from build123d import *

# Parameters (mm, degrees)
SKETCH010_W      = 209.545
SKETCH010_H      = 125
SKETCH010_R      = 1.6
EXTRUDE010_DEPTH = 1.6
SKETCH015_W      = 28
SKETCH015_H      = 8.6
EXTRUDE014_DEPTH = 10


with BuildPart() as extrude010:
    # Sketch010 → Extrude010 (new body)
    with BuildSketch(Plane.XY.offset(38)):
        with Locations((192.2275, 147.5)):
            Rectangle(SKETCH010_W, SKETCH010_H)
        with Locations((93.455, 204)):
            Circle(SKETCH010_R, mode=Mode.SUBTRACT)
        with Locations((291, 204)):
            Circle(SKETCH010_R, mode=Mode.SUBTRACT)
        with Locations((291, 91)):
            Circle(SKETCH010_R, mode=Mode.SUBTRACT)
        with Locations((93.455, 91)):
            Circle(SKETCH010_R, mode=Mode.SUBTRACT)
    extrude(amount=EXTRUDE010_DEPTH)


with BuildPart() as rf16:
    # Sketch015 (on Face10 of Extrude010) → Extrude014 (new body)
    with BuildSketch(Plane.XY.offset(39.6)):
        with Locations((272.87, 107.23)):
            Rectangle(SKETCH015_W, SKETCH015_H)
        with Locations((272.87, 117.39)):
            Rectangle(SKETCH015_W, SKETCH015_H)
        with Locations((208.11, 198.57)):
            Rectangle(SKETCH015_W, SKETCH015_H)
        with Locations((178.9, 198.57)):
            Rectangle(SKETCH015_W, SKETCH015_H)
        with Locations((149.69, 198.57)):
            Rectangle(SKETCH015_W, SKETCH015_H)
        with Locations((120.48, 198.57)):
            Rectangle(SKETCH015_W, SKETCH015_H)
    extrude(amount=EXTRUDE014_DEPTH)

    # Fusion005: union Extrude010
    add(extrude010.part)


solid = rf16.part
Source: CAD feature listing. Evaluate the final solid. Frame: model axes, mm. A direction names the side the tool comes from. Give positions to 0.01 mm unless a question says otherwise; leave off trailing zeros. Order: outer loops, then holes, each group sorted by start corner. A loop starts at its lowest first (then second) coordinate and runs counter-clockwise, first axis right, second up. Notation, with made-up numbers: (37.25, -20.5) -> (51.25, -20.5) arc R23 ccw to (51.25, 8.5) -> close; hole circle Ø3 at (88.25, -18.75). An arc over 180 degrees is marked (long way). Use a Markdown table: item, result.
1) Ray query, line 1 along X through (y, z) = (204, 38.4) (3 decimals); line 2 along X through (y, z) = (197.5, 43); line 3 along Y through (x, z) = (291, 38.75). Return the intervals inside material, ascending. Write a range as [from, to].
Answer list:
| item | result |
|---|---|
| line 1 | [87.455, 91.855], [95.055, 289.4], [292.6, 297] |
| line 2 | [106.48, 134.48], [135.69, 163.69], [164.9, 192.9], [194.11, 222.11] |
| line 3 | [85, 89.4], [92.6, 202.4], [205.6, 210] |
2) Section query A-A, the plane z = 42.5. Return the cut outline in (x, y).
Answer list:
| item | result |
|---|---|
| outline | (106.48, 194.27) -> (134.48, 194.27) -> (134.48, 202.87) -> (106.48, 202.87) -> close; (135.69, 194.27) -> (163.69, 194.27) -> (163.69, 202.87) -> (135.69, 202.87) -> close; (164.9, 194.27) -> (192.9, 194.27) -> (192.9, 202.87) -> (164.9, 202.87) -> close; (194.11, 194.27) -> (222.11, 194.27) -> (222.11, 202.87) -> (194.11, 202.87) -> close; (258.87, 102.93) -> (286.87, 102.93) -> (286.87, 111.53) -> (258.87, 111.53) -> close; (258.87, 113.09) -> (286.87, 113.09) -> (286.87, 121.69) -> (258.87, 121.69) -> close |
3) Contact query for flat-ended pins moving along their axis: P1, Ø1.5, axis at x = 146.5, z = 43, coming from the +Y side; P2, Ø3, axis at x = 291, y = 91, coming from the -Z side; P3, Ø2.5, axis at y = 199.5, z = 43, coming from the +X side; P4, Ø5, axis at x = 213.5, z = 43.5, coming from the -Y side. Output: stop coordinate, or through.
Answer list:
| item | result |
|---|---|
| P1 | y = 202.87 |
| P2 | through |
| P3 | x = 222.11 |
| P4 | y = 194.27 |
4) Reachability of faces 4 (the flat face through (286.87, 117, 45)), 5 (the flat face through (273, 111.53, 45)), 6 (the flat face through (164.9, 199, 45)), 7 (the flat face through (149, 202.87, 45)), 8 (the flat face through (208, 194.27, 45)) from +Z, -Z, +X, -X, +Y, -Y: full face, straight path, thin tool, end or side. Return the list, or none.
Answer list:
| item | result |
|---|---|
| face 4 | +Z, +X, +Y, -Y |
| face 5 | +Z, +X, -X |
| face 6 | +Z, +Y, -Y |
| face 7 | +Z, +X, -X, +Y |
| face 8 | +Z, +X, -X, -Y |
5) Section query D-D, the plane x = 255. Return the cut outline in (y, z), then the cut area to 3 significant figures.
Answer list:
| item | result |
|---|---|
| outline | (85, 38) -> (210, 38) -> (210, 39.6) -> (85, 39.6) -> close |
| area | 200 mm² |
6) Mould query, pull axis X, two halves, no side actions, for faces 1 (the flat face through (222.11, 199, 45)), 2 (the flat face through (194.11, 199, 45)), 3 (the flat face through (208, 199, 49.6)). Classes: +X half, -X half, draft (parallel to the pull), parting line (faces both ways), or undercut.
Answer list:
| item | result |
|---|---|
| face 1 | +X half |
| face 2 | undercut |
| face 3 | draft |
7) Section query B-B, the plane x = 150.5. Return the cut outline in (y, z).
Answer list:
| item | result |
|---|---|
| outline | (85, 38) -> (210, 38) -> (210, 39.6) -> (202.87, 39.6) -> (202.87, 49.6) -> (194.27, 49.6) -> (194.27, 39.6) -> (85, 39.6) -> close |
8) Section query C-C, the plane y = 108.5. Return the cut outline in (x, z) (3 decimals), then the cut area to 3 significant figures.
Answer list:
| item | result |
|---|---|
| outline | (87.455, 38) -> (297, 38) -> (297, 39.6) -> (286.87, 39.6) -> (286.87, 49.6) -> (258.87, 49.6) -> (258.87, 39.6) -> (87.455, 39.6) -> close |
| area | 615 mm² |
